from build123d import *

# Parameters (mm, degrees)
SKETCH_4_R           = 3.875
SKETCH_4_R_2         = 1.795
EXTRUDE_3_DEPTH      = 1.25
EXTRUDE_4_DEPTH      = 1.65
EXTRUDE_4_DEPTH_BACK = 2.9
SKETCH_1_R           = 3.875
SKETCH_1_R_2         = 1.795


with BuildPart() as part:
    # Sketch 4 → Extrude 3 (new body)
    # profile 1 of 3: a face of its own
    with BuildSketch(Plane.XY.offset(2.9)):
        with BuildLine():
            ThreePointArc((3.175, -8.746386407), (0, -7.594000789), (-3.175, -8.746386407))
            ThreePointArc((-3.175, -8.746386407), (-11.3, -4.948772024), (-3.175, -1.151157641))
            ThreePointArc((-3.175, -1.151157641), (0, -2.303543258), (3.175, -1.151157641))
            ThreePointArc((3.175, -1.151157641), (11.3, -4.948772024), (3.175, -8.746386407))
        make_face()
        with Locations((-6.35, -4.948772024)):
            Circle(SKETCH_4_R, mode=Mode.SUBTRACT)
        with Locations((6.35, -4.948772024)):
            Circle(SKETCH_4_R, mode=Mode.SUBTRACT)
    # profile 2 of 3: a face of its own
    with BuildSketch(Plane.XY.offset(2.9)):
        with Locations((-6.35, -4.948772024)):
            Circle(SKETCH_4_R)
        with Locations((-6.35, -4.948772024)):
            Circle(SKETCH_4_R_2, mode=Mode.SUBTRACT)
    # profile 3 of 3: a face of its own
    with BuildSketch(Plane.XY.offset(2.9)):
        with Locations((6.35, -4.948772024)):
            Circle(SKETCH_4_R)
        with Locations((6.35, -4.948772024)):
            Circle(SKETCH_4_R_2, mode=Mode.SUBTRACT)
    extrude(amount=-EXTRUDE_3_DEPTH)


with BuildPart() as body_2:
    # Mirror 6: mirrored copy
    add(part.part.mirror(Plane.XY))


with BuildPart() as part_1:
    add(part.part)

    add(body_2.part)  # Extrude 4 merges body 2
    # Sketch 1 → Extrude 4 (add, two sides: drawn at the far end of the back side and taken through both)
    # profile 1 of 2: a face of its own
    with BuildSketch(Plane.XY.offset(-EXTRUDE_4_DEPTH_BACK)):
        with Locations((-6.35, -4.948772024)):
            Circle(SKETCH_1_R)
        with Locations((-6.35, -4.948772024)):
            Circle(SKETCH_1_R_2, mode=Mode.SUBTRACT)
    # profile 2 of 2: a face of its own
    with BuildSketch(Plane.XY.offset(-EXTRUDE_4_DEPTH_BACK)):
        with Locations((6.35, -4.948772024)):
            Circle(SKETCH_1_R)
        with Locations((6.35, -4.948772024)):
            Circle(SKETCH_1_R_2, mode=Mode.SUBTRACT)
    extrude(amount=EXTRUDE_4_DEPTH + EXTRUDE_4_DEPTH_BACK)


solid = part_1.part
Could you check a few things on this model? Use its own coordinates, in mm. A direction names the side the tool comes from. Round coordinates to 2 decimals unless told otherwise and drop trailing zeros. Write each loop counter-clockwise with the first axis right and the second up, starting at its lowest first coordinate (ties: lowest second). Pieces come first, ordered by that corner, then holes. Notation, with made-up numbers: (-28.75, 20.25) - (-17.75, 20.25) arc R14 cw to (-17.75, 31.25) - close; hole circle Ø10 at (-25.75, 6). An arc over 180 degrees is marked (long way). Use a Markdown table: item, result.
Q1. For pin 1 (1 mm diameter, centred on y = -3.5, z = 2, fed in from -X); pin 2 (4.5 mm diameter, centred on x = 6.35, y = -4.95, fed in from -Z); pin 3 (1.5 mm diameter, centred on y = -7.5, z = -1.5, fed in from +X), each with a flat end and sliding along its axis, tell me the tip position at first contact or that it passes through.
Output values:
| item | result |
|---|---|
| pin 1 | x = -11.21 |
| pin 2 | z = -2.9 |
| pin 3 | x = 10.95 |
Q2. I want a section at A-A (x = -6.35). List the corners of the cut face in (y, z) for me, plus the area to 3 significant figures.
Output values:
| item | result |
|---|---|
| outline | (-9.9, -2.9) - (-6.74, -2.9) - (-6.74, 2.9) - (-9.9, 2.9) - (-9.9, 1.65) - (-8.82, 1.65) - (-8.82, -1.65) - (-9.9, -1.65) - close; (-3.15, -2.9) - (0, -2.9) - (0, -1.65) - (-1.07, -1.65) - (-1.07, 1.65) - (0, 1.65) - (0, 2.9) - (-3.15, 2.9) - close |
| area | 29.5 mm2 |
Q3. Please list where these lines run through material, in increasing order: L1, parallel to X at y = -5, z = -2.05; L2, parallel to Y at x = -6.35, z = -0.3; L3, parallel to Y at x = -6.35, z = 2.05.
Output values:
| item | result |
|---|---|
| L1 | -11.3 to -8.14, -4.56 to 4.56, 8.14 to 11.3 |
| L2 | -8.82 to -6.74, -3.15 to -1.07 |
| L3 | -9.9 to -6.74, -3.15 to 0 |
Q4. I want a section at D-D (z = -0.2). List the corners of the cut face in (x, y) for me (3 decimals).
Output values:
| item | result |
|---|---|
| outline | circle Ø7.75 at (-6.35, -4.949); circle Ø7.75 at (6.35, -4.949); hole circle Ø3.59 at (-6.35, -4.949); hole circle Ø3.59 at (6.35, -4.949) |
Q5. Thinking about a two-plate mould opening in X: for faces 1 (the flat face through (0, -5, 1.65)), 2 (the flat face through (0, -5, -2.9)), which applies, released by +X, released by -X, zero draft, split by the parting line, or undercut?
Output values:
| item | result |
|---|---|
| face 1 | undercut |
| face 2 | zero draft |
Q6. I want a section at B-B (y = -2.75). List the corners of the cut face in (x, z) for me.
Output values:
| item | result |
|---|---|
| outline | (-10.78, -2.9) - (10.78, -2.9) - (10.78, -1.65) - (9.54, -1.65) - (9.54, 1.65) - (10.78, 1.65) - (10.78, 2.9) - (-10.78, 2.9) - (-10.78, 1.65) - (-9.54, 1.65) - (-9.54, -1.65) - (-10.78, -1.65) - close; hole (-3.16, -1.65) - (3.16, -1.65) - (3.16, 1.65) - (-3.16, 1.65) - close |
Q7. I want a section at C-C (y = -5.5). List the corners of the cut face in (x, z) for me, plus the area to 3 significant figures.
Output values:
| item | result |
|---|---|
| outline | (-11.27, -2.9) - (-8.06, -2.9) - (-8.06, 2.9) - (-11.27, 2.9) - (-11.27, 1.65) - (-10.19, 1.65) - (-10.19, -1.65) - (-11.27, -1.65) - close; (-4.64, -2.9) - (4.64, -2.9) - (4.64, 2.9) - (-4.64, 2.9) - close; (8.06, -2.9) - (11.27, -2.9) - (11.27, -1.65) - (10.19, -1.65) - (10.19, 1.65) - (11.27, 1.65) - (11.27, 2.9) - (8.06, 2.9) - close; hole (-2.51, -1.65) - (2.51, -1.65) - (2.51, 1.65) - (-2.51, 1.65) - close |
| area | 67.3 mm2 |
Q8. For faces 3 (the cylindrical face through (-10.22, -4.78, -0.02)), 4 (the flat face through (0, -5, 2.9)), which set-ups out of +Z, -Z, +X, -X, +Y, -Y let a thin tool reach every point of the face, with its end or its side?
Output values:
| item | result |
|---|---|
| face 3 | none |
| face 4 | +Z, +X, -X, +Y, -Y |
